For this review, take the finished solid that the model builds, in its own axes (mm). A direction names the side the tool comes from. Round coordinates to 2 decimals unless told otherwise and drop trailing zeros. Order: outer loops, then holes, each group sorted by start corner. A loop starts at its lowest first (then second) coordinate and runs counter-clockwise, first axis right, second up. Notation, with made-up numbers: M 77.25,48 L 110.25,48 A18 ccw 110.25,67 Z; hole C -20,-16.75 d8. An arc over 180 degrees is marked long. Put each result on its own line as item: value.
from build123d import *

# Parameters (mm, degrees)
F0_W     = 800
F0_H     = 300
F1_DEPTH = 400
F2_R     = 40
F3_SIZE  = 30
F5_DEPTH = 5
F6_T     = 5
F8_DEPTH = 800.001


# Not quite as in the source:
# - a shell that OpenCascade refuses in one call is made with other operations: the cavity is built on its own and cut out


with BuildPart() as f1:
    # F0 (on Front) → F1 (new body)
    with BuildSketch(Plane.XZ):
        Rectangle(F0_W, F0_H)
    extrude(amount=F1_DEPTH)

    # F2
    f2_edges = [f1.edges().sort_by_distance(p)[0] for p in [
        (400, -200, 150),
        (-400, -200, 150),
        (400, -200, -150),
        (-400, -200, -150),
    ]]
    fillet(f2_edges, radius=F2_R)

    # F3
    f3_edges = [f1.edges().sort_by_distance(p)[0] for p in [
        (0, 0, 150),
        (0, 0, -150),
        (-388.284271, 0, -138.284271),
        (388.284271, 0, -138.284271),
        (-400, 0, 0),
        (400, 0, 0),
        (-388.284271, 0, 138.284271),
        (388.284271, 0, 138.284271),
    ]]
    chamfer(f3_edges, length=F3_SIZE)

    # F4 (on face) → F5 (cut)
    with BuildSketch(Plane(origin=(0, 0, 0), x_dir=(-1, 0, 0), z_dir=(0, 1, 0))):
        with BuildLine():
            Line((366.9999986887, -110), (366.9999986887, 110))
            ThreePointArc((366.9999986887, 110), (364.9497465411, 114.9497465411), (360, 116.9999986887))
            Line((360, 116.9999986887), (-360, 116.9999986887))
            ThreePointArc((-360, 116.9999986887), (-364.9497465411, 114.9497465411), (-366.9999986887, 110))
            Line((-366.9999986887, 110), (-366.9999986887, -110))
            ThreePointArc((-366.9999986887, -110), (-364.9497465411, -114.9497465411), (-360, -116.9999986887))
            Line((-360, -116.9999986887), (360, -116.9999986887))
            ThreePointArc((360, -116.9999986887), (364.9497465411, -114.9497465411), (366.9999986887, -110))
        make_face()
    extrude(amount=-F5_DEPTH, mode=Mode.SUBTRACT)

    # F6: shell of thickness 5, made by hand


with BuildPart() as f6_core1:
    # F6_t2: copy of F1
    add(f1.part)

    # the walls: a layer under each face that stays
    f6_faces = [f6_core1.faces().sort_by_distance(p)[0] for p in [
        (0, -215, -150),
        (-388.2842712475, -215, -138.2842712475),
        (0, -15, -135),
        (0, -400, 0),
        (388.2842712475, -215, -138.2842712475),
        (-377.6776695297, -15, -127.6776695297),
        (-400, -215, 0),
        (254.375, 0, -117.037037037),
        (377.6776695297, -15, -127.6776695297),
        (400, -215, 0),
        (-388.2842712475, -215, 138.2842712475),
        (388.2842712475, -215, 138.2842712475),
        (0, -215, 150),
        (-385, -15, 0),
        (0, -15, 135),
        (377.6776695297, -15, 127.6776695297),
        (-377.6776695297, -15, 127.6776695297),
        (385, -15, 0),
        (364.9497465411, -2.5, -114.9497465411),
        (366.9999986887, -2.5, 0),
        (364.9497465411, -2.5, 114.9497465411),
        (0, -2.5, 116.9999986887),
        (-364.9497465411, -2.5, 114.9497465411),
        (-366.9999986887, -2.5, 0),
        (-364.9497465411, -2.5, -114.9497465411),
        (0, -2.5, -116.9999986887),
    ]]
    thicken(f6_faces, amount=-F6_T, mode=Mode.SUBTRACT)


with BuildPart() as f1_1:
    add(f1.part)

    # what is left inside the walls is the cavity
    f6_cavity = [f6_core1.part.solids().sort_by_distance(p)[0] for p in [
        (0, -274.023689, -144.95),
    ]]
    add(f6_cavity, mode=Mode.SUBTRACT)

    # F7 (on face) → F8 (cut, through all)
    with BuildSketch(Plane.YZ.offset(400)):
        with BuildLine():
            Line((-375, -20), (-55, -20))
            ThreePointArc((-55, -20), (-51.4644660941, -18.5355339059), (-50, -15))
            Line((-50, -15), (-50, 15))
            ThreePointArc((-50, 15), (-51.4644660941, 18.5355339059), (-55, 20))
            Line((-55, 20), (-375, 20))
            ThreePointArc((-375, 20), (-378.5355339059, 18.5355339059), (-380, 15))
            Line((-380, 15), (-380, -15))
            ThreePointArc((-380, -15), (-378.5355339059, -18.5355339059), (-375, -20))
        make_face()
    extrude(amount=-F8_DEPTH, mode=Mode.SUBTRACT)


solid = f1_1.part
(1) Add section A-A on y = -274. Give the boundary of the cut face in (x, z), then the cut area to 3 significant figures.
A:
outline: M -400,-110 A40 ccw -360,-150 L 360,-150 A40 ccw 400,-110 L 400,-20 L 395,-20 L 395,-110 A35 cw 360,-145 L -360,-145 A35 cw -395,-110 L -395,-20 L -400,-20 Z; M -400,20 L -395,20 L -395,110 A35 cw -360,145 L 360,145 A35 cw 395,110 L 395,20 L 400,20 L 400,110 A40 ccw 360,150 L -360,150 A40 ccw -400,110 Z
area: 10,200 mm2
(2) Draft analysis for pull direction X (two halves, no side actions). For faces 1 (the face through (387.972, -217.59, -138.594)), 2 (the face through (-395, -211, -26)), 3 (the face through (-5, -212, -150)), state which applies: released by +X, released by -X, zero draft, split by the parting line, or undercut.
A:
face 1: released by +X
face 2: undercut
face 3: zero draft
(3) Insertion check: pin 1 Ø1.5 at (x, y) = (-70, -1.5) entering from -Z; pin 2 Ø4 at (x, z) = (-43, 46.5) entering from +Y; pin 3 Ø1.5 at (x, z) = (-397.5, 7.5) entering from +Y. Each pin has a flat end and moves straight along its axis. Give the tip position at first contact, or say it passes through.
A:
pin 1: stops at z = -122.25
pin 2: stops at y = -395
pin 3: stops at y = -26.75
(4) Add section B-B on x = -192.5. Give the boundary of the cut face in (y, z).
A:
outline: M -400,-150 L -30,-150 L 0,-120 L 0,-117 L -5,-117 L -5,-117.93 L -32.07,-145 L -395,-145 L -395,145 L -32.07,145 L -5,117.93 L -5,117 L 0,117 L 0,120 L -30,150 L -400,150 Z
(5) To check wall thickness, follow L1, parallel to Y at x = 122, z = -118; L2, parallel to X at y = -306, z = -34.5; L3, parallel to Z at x = 350, y = -213.5. State the ranges of each line that lie inside material, in increasing order.
A:
L1: y = -400 to -395, -5.07 to 0
L2: x = -400 to -395, 395 to 400
L3: z = -150 to -145, 145 to 150
(6) For faces 4 (the face through (-378.02, -15.21, 127.63)), 5 (the face through (375.479, -18.725, -125.142)), list the 3-axis set-ups (+Z, -Z, +X, -X, +Y, -Y) from which the entire face can be reached by the end or side of a thin tool; tool diameter is ignored.
A:
face 4: +Z, -X, +Y
face 5: none
(7) Add section C-C on z = 96. Give the boundary of the cut face in (x, y).
A:
outline: M -400,-400 L 400,-400 L 400,-30 L 370,0 L 367,0 L 367,-5 L 367.93,-5 L 395,-32.07 L 395,-395 L -395,-395 L -395,-32.07 L -367.93,-5 L -367,-5 L -367,0 L -370,0 L -400,-30 Z
